Check sheet for the modelled part. Datum: model origin and axes. Units: mm. A direction names the side the tool comes from. Coordinates: 2 decimals unless noted, no trailing zeros. Loops run counter-clockwise (first coordinate to the right, second up) from the corner with the lowest first, then second, coordinate; pieces in that order, holes last. Notation, with made-up numbers: M 75,48 L 117,48 A20 ccw 117,79 Z; hole C 47,89 d3. An arc over 180 degrees is marked long. Answer in a Markdown table with one row per item. Add a question column.
```python
from build123d import *

# Parameters (mm, degrees)
BOSS_EXTRUDE1_DEPTH = 15
SKETCH2_R           = 4.25
CUT_EXTRUDE1_DEPTH  = 69.260969814
SKETCH3_R           = 2
CUT_EXTRUDE2_DEPTH  = 7
CUT_EXTRUDE3_START  = -7
SKETCH4_R           = 2
CUT_EXTRUDE3_DEPTH  = 7
FILLET1_R           = 0.1


with BuildPart() as part:
    # Sketch1 → Boss-Extrude1 (new body)
    with BuildSketch(Plane(origin=(0, 0, 0), x_dir=(1, 0, 0), z_dir=(0, 1, 0))):
        Polygon((48.4, 32), (58.4, 32), (58.4, 0), (0, 0), (0, 32), (10, 32), (10, 10), (48.4, 10), align=None)
    extrude(amount=BOSS_EXTRUDE1_DEPTH)

    # Sketch2 → Cut-Extrude1 (cut, through all)
    with BuildSketch(Plane.ZY):
        with Locations((-25, 7.5)):
            Circle(SKETCH2_R)
    extrude(amount=-CUT_EXTRUDE1_DEPTH, mode=Mode.SUBTRACT)

    # Sketch3 → Cut-Extrude2 (cut)
    with BuildSketch(Plane.ZY):
        with Locations((-5, 7.5)):
            Circle(SKETCH3_R)
    extrude(amount=-CUT_EXTRUDE2_DEPTH, mode=Mode.SUBTRACT)

    # Sketch4 → Cut-Extrude3 (cut)
    with BuildSketch(Plane(origin=(58.4, 0, 0), x_dir=(0, 0, -1), z_dir=(1, 0, 0)).offset(CUT_EXTRUDE3_START)):
        with Locations(Location((5, 7.5, 0), (0, 0, 180))):
            Circle(SKETCH4_R)
    extrude(amount=CUT_EXTRUDE3_DEPTH, mode=Mode.SUBTRACT)

    # Fillet1
    fillet1_edges = [part.edges().sort_by_distance(p)[0] for p in [
        (58.4, 15, -16),
        (29.2, 0, 0),
        (0, 0, -16),
        (53.4, 15, -32),
        (0, 7.5, -32),
        (10, 7.5, -32),
        (10, 7.5, -10),
        (48.4, 7.5, -10),
        (48.4, 7.5, -32),
        (58.4, 7.5, -32),
        (58.4, 7.5, 0),
        (0, 7.5, 0),
        (48.4, 15, -21),
        (29.2, 15, -10),
        (10, 15, -21),
        (5, 15, -32),
        (0, 15, -16),
        (29.2, 15, 0),
        (5, 0, -32),
        (10, 0, -21),
        (29.2, 0, -10),
        (48.4, 0, -21),
        (53.4, 0, -32),
        (58.4, 0, -16),
    ]]
    fillet(fillet1_edges, radius=FILLET1_R)


solid = part.part
```
Q1. Thickness scan on L1, parallel to Y at x = 2.75, z = -5; L2, parallel to X at y = 2.5, z = -19; L3, parallel to Y at x = 54.75, z = -25. Record the ranges inside material, lowest first.
Q2. Cross-section at D-D (y = 12.75). Record the cut outline in (x, z), plus the area to 3 significant figures.
Q3. Mould release check, pull along X, two halves, no side actions. Record for faces 1 (the face through (48.4, 7, -18)), 2 (the face through (7, 8, -5)), 3 (the face through (53, 7, -32)), 4 (the face through (29, 7, -10)): released by +X, released by -X, zero draft, split by the parting line, or undercut.
Q4. Cross-section at B-B (y = 7.5). Count the separate pieces of the cut face and the enclosed holes in it, plus the area to 3 significant figures.
Q5. Go/stop test with flat-tipped pins: pin 1 (3 mm diameter, centred on y = 7.5, z = -5, fed in from -X); pin 2 (1.2 mm diameter, centred on y = 7, z = -5, fed in from +X); pin 3 (7.5 mm diameter, centred on x = 29, y = 8, fed in from -Z). Record where each tip stops, or that it passes through.
Q6. Access from +Z, -Z, +X, -X, +Y, -Y to the whole of each face (thin tool, end or side, straight path). Record for faces 5 (the face through (54.851, 6.148, -6.474)), 6 (the face through (3.451, 9.483, -5.26)), 7 (the face through (10, 7, -19)).
Q7. Cross-section at C-C (x = 4). Record the cut outline in (y, z), plus the area to 3 significant figures.
Q8. Cross-section at A-A (z = -25). Record the cut outline in (x, y), plus the area to 3 significant figures.
Answer key:
| question | item | result |
|---|---|---|
| 1 | L1 | 0 to 5.5, 9.5 to 15 |
| 1 | L2 | 0 to 10, 48.4 to 58.4 |
| 1 | L3 | 0 to 3.25, 11.75 to 15 |
| 2 | outline | M 0,-31.9 A0.1 ccw 0.1,-32 L 9.9,-32 A0.1 ccw 10,-31.9 L 10,-10.1 A0.1 cw 10.1,-10 L 48.3,-10 A0.1 cw 48.4,-10.1 L 48.4,-31.9 A0.1 ccw 48.5,-32 L 58.3,-32 A0.1 ccw 58.4,-31.9 L 58.4,-0.1 A0.1 ccw 58.3,0 L 0.1,0 A0.1 ccw 0,-0.1 Z |
| 2 | area | 1,020 mm^2 |
| 3 | face 1 | undercut |
| 3 | face 2 | released by -X |
| 3 | face 3 | zero draft |
| 3 | face 4 | undercut |
| 4 | separate pieces | 3 |
| 4 | enclosed holes | 0 |
| 4 | area | 798 mm^2 |
| 5 | pin 1 | x = 7 |
| 5 | pin 2 | x = 51.4 |
| 5 | pin 3 | z = -10 |
| 6 | face 5 | +X |
| 6 | face 6 | -X |
| 6 | face 7 | -Z, +Y, -Y |
| 7 | outline | M 0,-31.9 A0.1 ccw 0.1,-32 L 14.9,-32 A0.1 ccw 15,-31.9 L 15,-0.1 A0.1 ccw 14.9,0 L 0.1,0 A0.1 ccw 0,-0.1 Z; hole C 7.5,-25 d8.5; hole C 7.5,-5 d4 |
| 7 | area | 411 mm^2 |
| 8 | outline | M 0,0.1 A0.1 ccw 0.1,0 L 9.9,0 A0.1 ccw 10,0.1 L 10,3.25 L 0,3.25 Z; M 0,11.75 L 10,11.75 L 10,14.9 A0.1 ccw 9.9,15 L 0.1,15 A0.1 ccw 0,14.9 Z; M 48.4,0.1 A0.1 ccw 48.5,0 L 58.3,0 A0.1 ccw 58.4,0.1 L 58.4,3.25 L 48.4,3.25 Z; M 48.4,11.75 L 58.4,11.75 L 58.4,14.9 A0.1 ccw 58.3,15 L 48.5,15 A0.1 ccw 48.4,14.9 Z |
| 8 | area | 130 mm^2 |
